from build123d import *

# Parameters (mm, degrees)
SKETCH1_W           = 35
SKETCH1_H           = 35
BOSS_EXTRUDE1_DEPTH = 5
SKETCH2_W           = 25.5
SKETCH2_H           = 25.5
SKETCH2_W_2         = 20.5
SKETCH2_H_2         = 20.5
BOSS_EXTRUDE2_DEPTH = 20
FILLET1_R           = 7.25
FILLET2_R           = 2.5


with BuildPart() as part:
    # Sketch1 → Boss-Extrude1 (new body)
    with BuildSketch(Plane(origin=(0, 0, 0), x_dir=(1, 0, 0), z_dir=(0, 1, 0))):
        with Locations((-10.693342281, -7.01463487)):
            Rectangle(SKETCH1_W, SKETCH1_H)
    extrude(amount=BOSS_EXTRUDE1_DEPTH)

    # Sketch2 → Boss-Extrude2 (add)
    with BuildSketch(Plane(origin=(0, 5, 0), x_dir=(1, 0, 0), z_dir=(0, 1, 0))):
        with Locations((-10.693342281, -7.01463487)):
            Rectangle(SKETCH2_W, SKETCH2_H)
        with Locations((-10.693342281, -7.01463487)):
            Rectangle(SKETCH2_W_2, SKETCH2_H_2, mode=Mode.SUBTRACT)
    extrude(amount=BOSS_EXTRUDE2_DEPTH)

    # Fillet1
    fillet1_edges = [part.edges().sort_by_distance(p)[0] for p in [
        (6.806657719, 2.5, 24.51463487),
        (-28.193342281, 2.5, 24.51463487),
        (-28.193342281, 2.5, -10.48536513),
        (6.806657719, 2.5, -10.48536513),
    ]]
    fillet(fillet1_edges, radius=FILLET1_R)

    # Fillet2
    fillet2_edges = [part.edges().sort_by_distance(p)[0] for p in [
        (-23.443342281, 15, -5.73536513),
        (-23.443342281, 15, 19.76463487),
        (2.056657719, 15, 19.76463487),
        (2.056657719, 15, -5.73536513),
    ]]
    fillet(fillet2_edges, radius=FILLET2_R)


solid = part.part
Input: part model. Units: mm. Frame: model coordinates. A direction names the side the tool comes from. Give positions to 0.01 mm unless a question says otherwise; leave off trailing zeros. Loops run counter-clockwise (first coordinate to the right, second up) from the corner with the lowest first, then second, coordinate; pieces in that order, holes last. Notation, with made-up numbers: M 10,-19 L 31,-19 A18 cw 31,-6 Z; hole C 4,63 d5. An arc over 180 degrees is marked long. Use CSV: the item, a comma, the result in double quotes.
(1) Section A-A, the plane y = 11.5. Return loops of the section in (x, z).
Outcome:
outline,"M -23.44,-3.24 A2.5 ccw -20.94,-5.74 L -0.44,-5.74 A2.5 ccw 2.06,-3.24 L 2.06,17.26 A2.5 ccw -0.44,19.76 L -20.94,19.76 A2.5 ccw -23.44,17.26 Z; hole M -20.94,-3.24 L -0.44,-3.24 L -0.44,17.26 L -20.94,17.26 Z"
(2) Pull-direction query (Z, two-part tool) for faces 6 (the face through (-20.943, 15, 7)), 7 (the face through (-26.126, 2.535, -8.305)), 8 (the face through (4.627, 2.535, 22.447)), 9 (the face through (-28.193, 2, 7)); classes: pulls with the +Z half, pulls with the -Z half, needs draft (parallel to the pull), parting line crosses it, or undercut.
Outcome:
face 6,"undercut"
face 7,"pulls with the -Z half"
face 8,"pulls with the +Z half"
face 9,"needs draft"
(3) Section C-C, the plane x = -5.5. Return loops of the section in (y, z).
Outcome:
outline,"M 0,-10.49 L 5,-10.49 L 5,-5.74 L 25,-5.74 L 25,-3.24 L 5,-3.24 L 5,17.26 L 25,17.26 L 25,19.76 L 5,19.76 L 5,24.51 L 0,24.51 Z"
(4) Set-up query: faces 1 (the face through (-23.443, 15, 7)), 2 (the face through (-11, 15, -3.235)), 3 (the face through (-11, 2, 24.515)), 4 (the face through (-22.692, 15.14, -5.022)), 5 (the face through (1.344, 15.14, -4.984)). Return all of +Z, -Z, +X, -X, +Y, -Y with unobstructed straight access to the full face (end or side cutting, diameter ignored); none if empty.
Outcome:
face 1,"+Z, -Z, -X, +Y"
face 2,"+Y"
face 3,"+Z, +X, -X, +Y, -Y"
face 4,"-Z, -X, +Y"
face 5,"-Z, +X, +Y"
(5) Pin query (flat end, axial travel): P1, Ø2, axis at x = -0.5, y = 7, coming from the +Z side; P2, Ø6, axis at y = 12.5, z = 7, coming from the +X side; P3, Ø10, axis at x = -12.5, y = 16.5, coming from the -Z side. Return the tip coordinate at first contact, or that it passes through.
Outcome:
P1,"stops at z = 19.76"
P2,"stops at x = 2.06"
P3,"stops at z = -5.74"
(6) Material intervals for L1, parallel to X at y = 15.25, z = 6; L2, parallel to Z at x = -0.5, y = 15.5; L3, parallel to Y at x = -19.5, z = 13.5, sorted ascending. Write a range as [from, to].
Outcome:
L1,"x = [-23.44, -20.94], [-0.44, 2.06]"
L2,"z = [-5.74, -3.24], [17.26, 19.76]"
L3,"y = [0, 5]"
(7) Section B-B, the plane z = 16. Return loops of the section in (x, y).
Outcome:
outline,"M -28.19,0 L 6.81,0 L 6.81,5 L 2.06,5 L 2.06,25 L -0.44,25 L -0.44,5 L -20.94,5 L -20.94,25 L -23.44,25 L -23.44,5 L -28.19,5 Z"
